The listing builds one solid part. Answer for the finished solid, in the listing's coordinates (mm). A direction names the side the tool comes from. Give positions to 0.01 mm unless a question says otherwise; leave off trailing zeros. Loops run counter-clockwise (first coordinate to the right, second up) from the corner with the lowest first, then second, coordinate; pieces in that order, holes last. Notation, with made-up numbers: M -30,49.5 L 1,49.5 A13 cw 1,66.5 Z; hole C -38,-14 d5. An arc over 180 degrees is marked long. One line per item, written item: value. Start each with the question number.
Q1. A cutting plane is placed at A-A, the plane z = 7.75. Determine the outline of the cut face in (x, y), and give its area (3 significant figures).
Q2. For faces 1 (the flat face through (-6, -30, 8)), 2 (the flat face through (-9, -30, 3)), 3 (the flat face through (10, -30, -6)), determine the directions among +Z, -Z, +X, -X, +Y, -Y from which every point of the face is accessible in a straight line to the end or side of a thin tool.
Q3. Flat-ended cylindrical pins translate along their axes: pin 1 (2 mm diameter, centred on x = -0.5, y = -31, fed in from -Z); pin 2 (1.5 mm diameter, centred on x = 1, z = -7.5, fed in from -Y). Find the tip coordinate at first contact, or state that the pin passes through.
Q4. A cutting plane is placed at B-B, the plane z = 5.25. Determine the outline of the cut face in (x, y), and give its area (3 significant figures).
Q5. Consider L1, parallel to X at y = -14.5, z = -7.5; L2, parallel to X at y = -4.5, z = 9; L3, parallel to X at y = -31, z = 3.25. Determine where each line is inside the solid, lowest interval first.
Q6. The mould has two halves that part along Z. Classify faces 4 (the cylindrical face through (9.715, -29.58, 9.699)), 5 (the cylindrical face through (-9.715, -29.58, -9.699)), 6 (the flat face through (-5, -30, -8.5)): +Z half, -Z half, draft (parallel to the pull), parting line (faces both ways), or undercut.
from build123d import *

# Parameters (mm, degrees)
PAD_DEPTH          = 60
POCKET_DEPTH       = 380
POLARPATTERN_COUNT = 4
POCKET001_DEPTH    = 380


with BuildPart() as part:
    # Sketch → Pad (new body)
    with BuildSketch(Plane.XZ):
        with BuildLine():
            Line((-9, 10), (9, 10))
            ThreePointArc((10, 9), (9.707107, 9.707107), (9, 10))
            Line((10, 9), (10, -9))
            ThreePointArc((9, -10), (9.707107, -9.707107), (10, -9))
            Line((9, -10), (-9, -10))
            ThreePointArc((-10, -9), (-9.707107, -9.707107), (-9, -10))
            Line((-10, -9), (-10, 9))
            ThreePointArc((-9, 10), (-9.707107, 9.707107), (-10, 9))
        make_face()
    extrude(amount=PAD_DEPTH)

    # Sketch001 (on Face10 of Pad) → Pocket (cut)
    with BuildSketch(Plane.XZ.offset(60)):
        Polygon((-3.4, 10), (-3.4, 9.6), (-3, 9.6), (-3, 8.5), (-6, 8.5), (-6, 7), (-3.35, 4.7), (-0.65, 4.7), (0, 4.3), (0.65, 4.7), (3.35, 4.7), (6, 7), (6, 8.5), (3, 8.5), (3, 9.6), (3.4, 9.6), (3.4, 10), align=None)
    pocket = extrude(amount=-POCKET_DEPTH, mode=Mode.SUBTRACT)

    # PolarPattern: Pocket ×4 about axis
    polarpattern_axis = Axis((0, -60, 0), (0, -1, 0))
    for i in range(1, POLARPATTERN_COUNT):
        add(pocket.rotate(polarpattern_axis, i * 360 / POLARPATTERN_COUNT), mode=Mode.SUBTRACT)

    # Sketch002 (on Face4 of PolarPattern) → Pocket001 (cut)
    with BuildSketch(Plane.XZ.offset(60)):
        with BuildLine():
            ThreePointArc((1.340499, 2.401159), (0, 2.75), (-1.340499, 2.401159))
            Line((-1.944544, 3.005204), (-1.340499, 2.401159))
            Line((-3.005204, 1.944544), (-1.944544, 3.005204))
            Line((-2.401159, 1.340499), (-3.005204, 1.944544))
            ThreePointArc((-2.401159, 1.340499), (-2.75, 0), (-2.401159, -1.340499))
            Line((-3.005204, -1.944544), (-2.401159, -1.340499))
            Line((-1.944544, -3.005204), (-3.005204, -1.944544))
            Line((-1.340499, -2.401159), (-1.944544, -3.005204))
            ThreePointArc((-1.340499, -2.401159), (0, -2.75), (1.340499, -2.401159))
            Line((1.944544, -3.005204), (1.340499, -2.401159))
            Line((3.005204, -1.944544), (1.944544, -3.005204))
            Line((2.401159, -1.340499), (3.005204, -1.944544))
            ThreePointArc((2.401159, -1.340499), (2.75, 0), (2.401159, 1.340499))
            Line((2.401159, 1.340499), (3.005204, 1.944544))
            Line((3.005204, 1.944544), (1.944544, 3.005204))
            Line((1.944544, 3.005204), (1.340499, 2.401159))
        make_face()
    extrude(amount=-POCKET001_DEPTH, mode=Mode.SUBTRACT)


solid = part.part
Answer block:
1. outline: M -10,-60 L -6,-60 L -6,0 L -10,0 Z; M 6,-60 L 10,-60 L 10,0 L 6,0 Z
1. area: 480 mm^2
2. face 1: +Y, -Y
2. face 2: -X, +Y, -Y
2. face 3: +Z, -Z, +X, +Y, -Y
3. pin 1: z = -4.7
3. pin 2: through
4. outline: M -10,-60 L -8.5,-60 L -8.5,0 L -10,0 Z; M -6.35,-60 L -3.98,-60 L -3.98,0 L -6.35,0 Z; M 3.98,-60 L 6.35,-60 L 6.35,0 L 3.98,0 Z; M 8.5,-60 L 10,-60 L 10,0 L 8.5,0 Z
4. area: 464 mm^2
5. L1: -10 to -6, 6 to 10
5. L2: -10 to -3, 3 to 10
5. L3: -9.6 to -8.5, -4.7 to 4.7, 8.5 to 9.6
6. face 4: +Z half
6. face 5: -Z half
6. face 6: undercut
